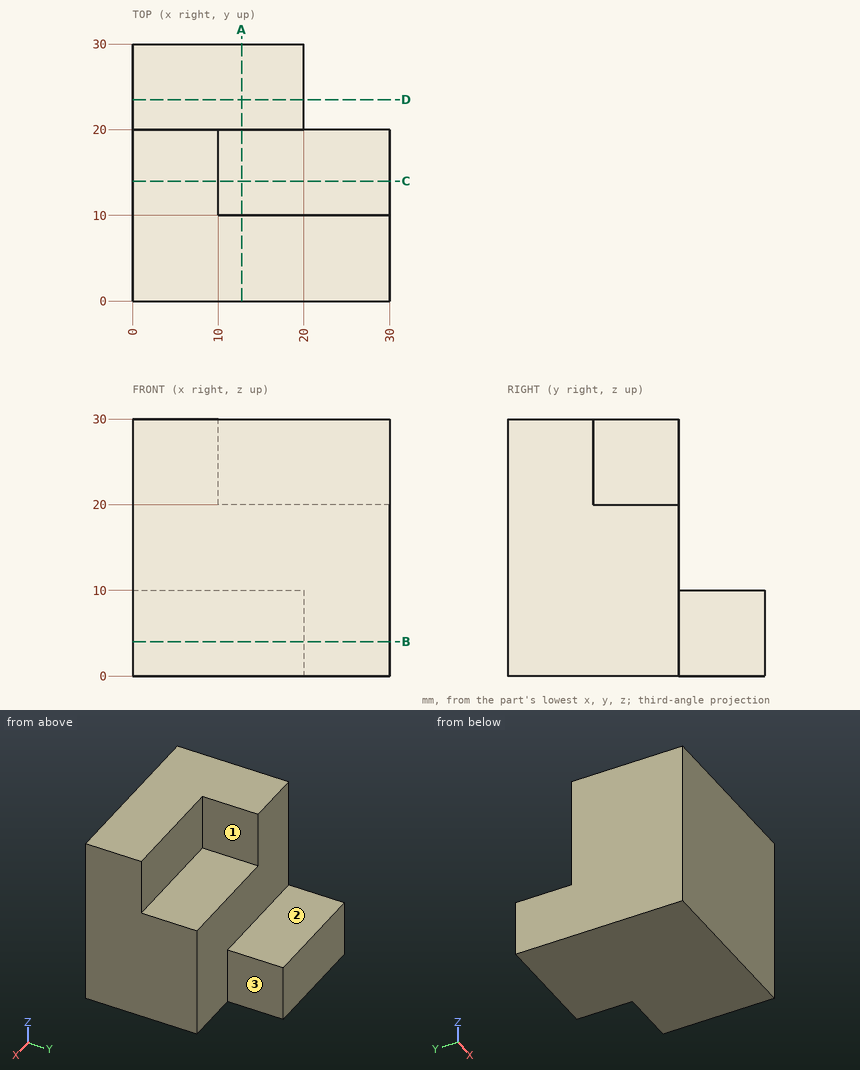
Design review of the part shown in the three views and the two pictorial views. Dimensions are in mm from the part's minimum x, y and z. A direction names the side the tool comes from. Give positions to 0.01 mm unless a question says otherwise; leave off trailing zeros. Write each loop counter-clockwise with the first axis right and the second up, starting at its lowest first coordinate (ties: lowest second). Pieces come first, ordered by that corner, then holes. Notation, with made-up numbers: (-21, 49) - (-6, 49) arc R26 ccw to (-6, 78) - close; hole circle Ø1 at (19, 75.5). An arc over 180 degrees is marked (long way). Return JSON: item names as keys, results as strings. Group by question number.
(1) Machinability: for the marked faces 1, 2 and 3, which of the approach directions +Z, -Z, +X, -X, +Y, -Y give a long, thin tool a straight path to every point of the face, cutting with its end or side? Answer none if there is none.
(2) Insertion check: pin 1 (6 mm diameter, centred on y = 25.5, z = 14, fed in from -X); pin 2 (5 mm diameter, centred on y = 26, z = 4, fed in from +X); pin 3 (2 mm diameter, centred on x = 23.5, z = 9, fed in from +Y); pin 4 (4 mm diameter, centred on x = 14.5, y = 25.5, fed in from +Z). Each pin has a flat end and moves straight along its axis. Give the tip position at first contact, or say it passes through.
(3) We need section A-A, the plane x = 12.75. Give the boundary of the cut face in (y, z), then the cut area to 3 significant figures.
(4) To check wall thickness, follow probe 1 along Y at (x, z) = (2, 13); probe 2 along Y at (x, z) = (11.75, 27). State the ranges of each line that lie inside material, in increasing order.
(5) We need section B-B, the plane z = 4. Give the boundary of the cut face in (x, y).
(6) We need section D-D, the plane y = 23.5. Give the boundary of the cut face in (x, z).
(7) We need section C-C, the plane y = 14. Give the boundary of the cut face in (x, z), then the cut area to 3 significant figures.
Reported:
{
 "1": {"face 1": "+Z, +X, +Y", "face 2": "+Z, +X, -X, +Y", "face 3": "+Z, -Z, +X, +Y"},
 "2": {"pin 1": "passes through", "pin 2": "stops at x = 20", "pin 3": "stops at y = 20", "pin 4": "stops at z = 10"},
 "3": {"outline": "(0, 0) - (30, 0) - (30, 10) - (20, 10) - (20, 20) - (10, 20) - (10, 30) - (0, 30) - close", "area": "600 mm2"},
 "4": {"probe 1": "y = 0 to 20", "probe 2": "y = 0 to 10"},
 "5": {"outline": "(0, 0) - (30, 0) - (30, 20) - (20, 20) - (20, 30) - (0, 30) - close"},
 "6": {"outline": "(0, 0) - (20, 0) - (20, 10) - (0, 10) - close"},
 "7": {"outline": "(0, 0) - (30, 0) - (30, 20) - (10, 20) - (10, 30) - (0, 30) - close", "area": "700 mm2"}
}
